Can you work these out from the drawing? Everything is in mm from the part's minimum corner. Round coordinates to 2 decimals unless told otherwise and drop trailing zeros. Order: outer loops, then holes, each group sorted by start corner. A loop starts at its lowest first (then second) coordinate and runs counter-clockwise, first axis right, second up. Notation, with made-up numbers: (88.5, 50) -> (107.5, 50) arc R28 ccw to (107.5, 86) -> close; hole circle Ø2 at (53.5, -28.5). An arc over 180 degrees is marked (long way). Use a Markdown table: item, result. Add a question column.
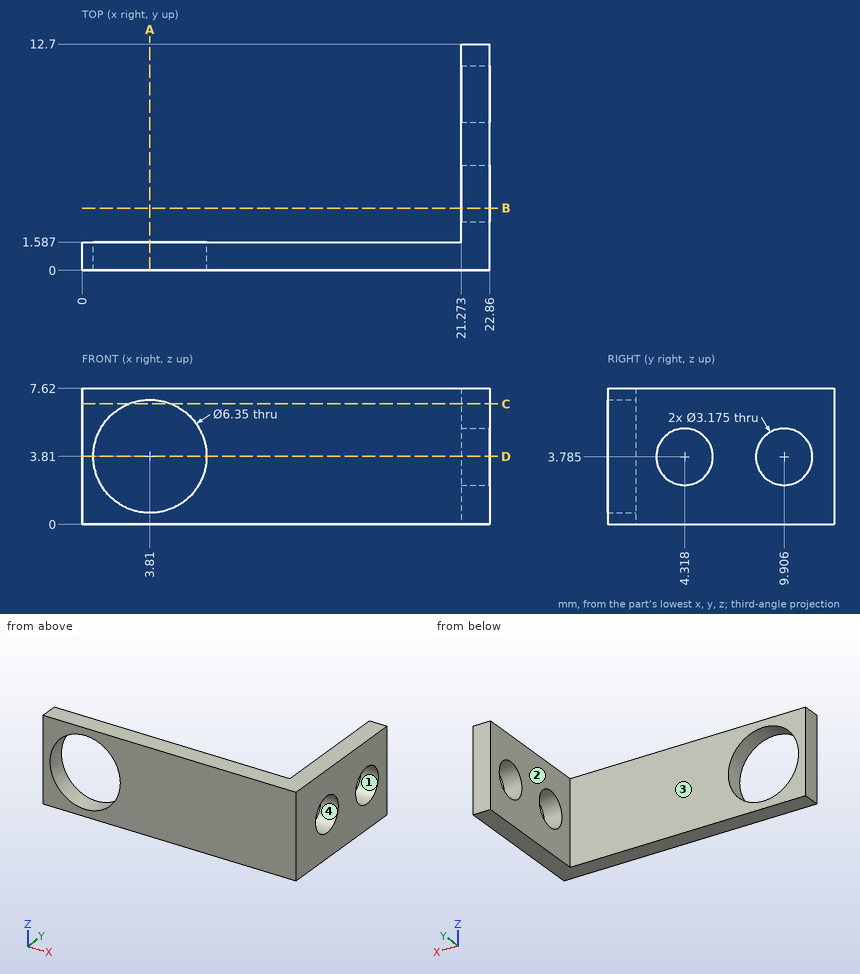
(1) If we mould it in two halves opening along Y, with no side actions, what happens to the marked faces 1, 2, 3 and 4? For each: pulls with the +Y half, pulls with the -Y half, needs draft (parallel to the pull), parting line crosses it, or undercut.
(2) I want a section at B-B on y = 3.5. List the corners of the cut face in (x, z) for me (1 decimal).
(3) I want a section at A-A on x = 3.81. List the corners of the cut face in (y, z) for me (1 decimal).
(4) I want a section at D-D on z = 3.81. List the corners of the cut face in (x, y) for me (1 decimal).
(5) I'm going to push flat-ended pins straight in: P1, Ø2.5, axis at x = 7, z = 2.5, coming from the +Y side; P2, Ø2, axis at x = 7, y = 4.5, coming from the -Z side; P3, Ø1.5, axis at y = 9.5, z = 1, coming from the -X side; P4, Ø2, axis at x = 20.5, y = 10.5, coming from the +Z side. Where does each tip first touch, or does it pass through?
(6) Please list where these lines run through material, in increasing order: probe 1 along Z at (x, y) = (3.81, 1) (1 decimal); probe 2 along Y at (x, z) = (21, 5.25); probe 3 along X at (y, z) = (6, 3). Write a range as from..to.
(7) I want a section at C-C on z = 6.75. List the corners of the cut face in (x, y) for me.
Output:
| question | item | result |
|---|---|---|
| 1 | face 1 | undercut |
| 1 | face 2 | needs draft |
| 1 | face 3 | pulls with the +Y half |
| 1 | face 4 | undercut |
| 2 | outline | (21.3, 0) -> (22.9, 0) -> (22.9, 2.4) -> (21.3, 2.4) -> close; (21.3, 5.1) -> (22.9, 5.1) -> (22.9, 7.6) -> (21.3, 7.6) -> close |
| 3 | outline | (0, 0) -> (1.6, 0) -> (1.6, 0.6) -> (0, 0.6) -> close; (0, 7) -> (1.6, 7) -> (1.6, 7.6) -> (0, 7.6) -> close |
| 4 | outline | (0, 0) -> (0.6, 0) -> (0.6, 1.6) -> (0, 1.6) -> close; (7, 0) -> (22.9, 0) -> (22.9, 2.7) -> (21.3, 2.7) -> (21.3, 1.6) -> (7, 1.6) -> close; (21.3, 5.9) -> (22.9, 5.9) -> (22.9, 8.3) -> (21.3, 8.3) -> close; (21.3, 11.5) -> (22.9, 11.5) -> (22.9, 12.7) -> (21.3, 12.7) -> close |
| 5 | P1 | y = 1.59 |
| 5 | P2 | through |
| 5 | P3 | x = 21.27 |
| 5 | P4 | z = 7.62 |
| 6 | probe 1 | 0..0.6, 7..7.6 |
| 6 | probe 2 | 0..1.59 |
| 6 | probe 3 | 21.27..22.86 |
| 7 | outline | (0, 0) -> (2.61, 0) -> (2.61, 1.59) -> (0, 1.59) -> close; (5.01, 0) -> (22.86, 0) -> (22.86, 12.7) -> (21.27, 12.7) -> (21.27, 1.59) -> (5.01, 1.59) -> close |
